from build123d import *

# Parameters (mm, degrees)
SKETCH1_W               = 61.1
SKETCH1_H               = 60
BOSS_EXTRUDE1_DEPTH     = 5
BOSS_EXTRUDE2_DEPTH     = 24
MIRROR2_COPY_1_DEPTH    = 24
SKETCH3_R               = 1.75
CUT_EXTRUDE1_DEPTH      = 60.592417722
MIRROR4_COPY_1_SKETCH_R = 1.75
MIRROR4_COPY_1_DEPTH    = 60.592417722
MIRROR5_COPY_1_SKETCH_R = 1.75
MIRROR5_COPY_1_DEPTH    = 60.592417722
MIRROR5_COPY_2_SKETCH_R = 1.75
MIRROR5_COPY_2_DEPTH    = 60.592417722
MIRROR5_COPY_3_SKETCH_R = 1.75
MIRROR5_COPY_3_DEPTH    = 60.592417722
SKETCH10_R              = 1.55
CUT_EXTRUDE7_DEPTH      = 8
SKETCH11_R              = 3
CUT_EXTRUDE8_DEPTH      = 1
SKETCH12_W              = 2
SKETCH12_H              = 30
SKETCH12_W_2            = 4
BOSS_EXTRUDE5_DEPTH     = 6.5
FILLET1_R               = 5
SKETCH12_4_W            = 0.75
SKETCH12_4_H            = 1
BOSS_EXTRUDE6_DEPTH     = 6.5
LPATTERN1_COUNT         = 15
LPATTERN1_PITCH         = 2
SKETCH13_R              = 1.55
CUT_EXTRUDE9_DEPTH      = 6.5


with BuildPart() as part:
    # Sketch1 → Boss-Extrude1 (new body)
    with BuildSketch(Plane(origin=(0, 0, 0), x_dir=(1, 0, 0), z_dir=(0, 1, 0))):
        Rectangle(SKETCH1_W, SKETCH1_H)
    extrude(amount=BOSS_EXTRUDE1_DEPTH)

    # Sketch2 → Boss-Extrude2 (add)
    with BuildSketch(Plane.XY.offset(30)):
        with BuildLine():
            Line((-30.55, 15.75), (-30.55, 5))
            Line((-30.55, 5), (-13.45, 5))
            Line((-13.45, 5), (-13.45, 15.75))
            Line((-13.45, 15.75), (-14.45, 15.75))
            ThreePointArc((-14.45, 15.75), (-22, 8.2), (-29.55, 15.75))
            Line((-29.55, 15.75), (-30.55, 15.75))
        make_face()
    boss_extrude2 = extrude(amount=-BOSS_EXTRUDE2_DEPTH)

    # Mirror1: Boss-Extrude2 across plane
    add(boss_extrude2.mirror(Plane.XY))

    # Mirror2: Boss-Extrude2 across plane
    add(boss_extrude2.mirror(Plane(origin=(0, 0, 0), x_dir=(0, 0, 1), z_dir=(1, 0, 0))))

    # Mirror2 copy 1 sketch → Mirror2 copy 1 (add)
    with BuildSketch(Plane(origin=(0, 0, -30), x_dir=(-1, 0, 0), z_dir=(0, 0, -1))):
        with BuildLine():
            Line((-30.55, 15.75), (-30.55, 5))
            Line((-30.55, 5), (-13.45, 5))
            Line((-13.45, 5), (-13.45, 15.75))
            Line((-13.45, 15.75), (-14.45, 15.75))
            ThreePointArc((-14.45, 15.75), (-22, 8.2), (-29.55, 15.75))
            Line((-29.55, 15.75), (-30.55, 15.75))
        make_face()
    extrude(amount=-MIRROR2_COPY_1_DEPTH)

    # Sketch3 → Cut-Extrude1 (cut, symmetric)
    with BuildSketch(Plane(origin=(-17.775, 17.775, 0), x_dir=(0.7071067811865477, 0.7071067811865475, 0), z_dir=(-0.7071067811865475, 0.7071067811865477, 0))):
        with Locations(Location((-13.965180362, -18, 0), (0, 0, 180))):
            Circle(SKETCH3_R)
    cut_extrude1 = extrude(amount=CUT_EXTRUDE1_DEPTH, both=True, mode=Mode.SUBTRACT)

    # Mirror3: Cut-Extrude1 across plane
    add(cut_extrude1.mirror(Plane.ZY.offset(22)), mode=Mode.SUBTRACT)

    # Mirror4: Cut-Extrude1 across plane
    add(cut_extrude1.mirror(Plane.XY), mode=Mode.SUBTRACT)

    # Mirror4 copy 1 sketch → Mirror4 copy 1 (cut, symmetric)
    with BuildSketch(Plane(origin=(-26.225, 17.775, 0), x_dir=(-0.7071067811865477, 0.7071067811865475, 0), z_dir=(0.7071067811865475, 0.7071067811865477, 0))):
        with Locations(Location((-13.965180362, -18, 0), (0, 0, 180))):
            Circle(MIRROR4_COPY_1_SKETCH_R)
    extrude(amount=MIRROR4_COPY_1_DEPTH, both=True, mode=Mode.SUBTRACT)

    # Mirror5: Cut-Extrude1 across plane
    add(cut_extrude1.mirror(Plane(origin=(0, 0, 0), x_dir=(0, 0, 1), z_dir=(1, 0, 0))), mode=Mode.SUBTRACT)

    # Mirror5 copy 1 sketch → Mirror5 copy 1 (cut, symmetric)
    with BuildSketch(Plane(origin=(26.225, 17.775, 0), x_dir=(0.7071067811865477, 0.7071067811865475, 0), z_dir=(-0.7071067811865475, 0.7071067811865477, 0))):
        with Locations(Location((-13.965180362, -18, 0), (0, 0, 180))):
            Circle(MIRROR5_COPY_1_SKETCH_R)
    extrude(amount=MIRROR5_COPY_1_DEPTH, both=True, mode=Mode.SUBTRACT)

    # Mirror5 copy 2 sketch → Mirror5 copy 2 (cut, symmetric)
    with BuildSketch(Plane(origin=(17.775, 17.775, 0), x_dir=(-0.7071067811865477, 0.7071067811865475, 0), z_dir=(0.7071067811865475, 0.7071067811865477, 0))):
        with Locations(Location((-13.965180362, -18, 0), (0, 0, 180))):
            Circle(MIRROR5_COPY_2_SKETCH_R)
    extrude(amount=MIRROR5_COPY_2_DEPTH, both=True, mode=Mode.SUBTRACT)

    # Mirror5 copy 3 sketch → Mirror5 copy 3 (cut, symmetric)
    with BuildSketch(Plane(origin=(26.225, 17.775, 0), x_dir=(0.7071067811865477, 0.7071067811865475, 0), z_dir=(-0.7071067811865475, 0.7071067811865477, 0))):
        with Locations((-13.965180362, 18)):
            Circle(MIRROR5_COPY_3_SKETCH_R)
    extrude(amount=MIRROR5_COPY_3_DEPTH, both=True, mode=Mode.SUBTRACT)

    # Sketch10 → Cut-Extrude7 (cut)
    with BuildSketch(Plane(origin=(0, 5, 0), x_dir=(1, 0, 0), z_dir=(0, 1, 0))):
        with Locations(Location((-6.45, -26, 0), (0, 0, 270))):
            Circle(SKETCH10_R)
        with Locations(Location((-6.45, 26, 0), (0, 0, 270))):
            Circle(SKETCH10_R)
        with Locations(Location((6.45, 26, 0), (0, 0, 270))):
            Circle(SKETCH10_R)
        with Locations(Location((6.45, -26, 0), (0, 0, 270))):
            Circle(SKETCH10_R)
    extrude(amount=-CUT_EXTRUDE7_DEPTH, mode=Mode.SUBTRACT)

    # Sketch11 → Cut-Extrude8 (cut)
    with BuildSketch(Plane.XZ):
        with Locations(Location((-6.45, 26, 0), (0, 0, 270))):
            Circle(SKETCH11_R)
        with Locations(Location((6.45, 26, 0), (0, 0, 270))):
            Circle(SKETCH11_R)
        with Locations(Location((6.45, -26, 0), (0, 0, 270))):
            Circle(SKETCH11_R)
        with Locations(Location((-6.45, -26, 0), (0, 0, 270))):
            Circle(SKETCH11_R)
    extrude(amount=-CUT_EXTRUDE8_DEPTH, mode=Mode.SUBTRACT)

    # Sketch12 → Boss-Extrude5 (add)
    with BuildSketch(Plane(origin=(0, 5, 0), x_dir=(1, 0, 0), z_dir=(0, 1, 0))):
        with Locations((-13.45, 0)):
            Rectangle(SKETCH12_W, SKETCH12_H)
        with Locations((-8.85, 0)):
            Rectangle(SKETCH12_W_2, SKETCH12_H)
    extrude(amount=BOSS_EXTRUDE5_DEPTH)

    # Fillet1
    fillet1_edges = [part.edges().sort_by_distance(p)[0] for p in [
        (-8.85, 5, 15),
        (-6.85, 5, 0),
        (-8.85, 5, -15),
        (-12.95, 5, -15),
        (-14.45, 5, 0),
        (-12.95, 5, 15),
    ]]
    fillet(fillet1_edges, radius=FILLET1_R)

    # Sketch12_4 → Boss-Extrude6 (add)
    with BuildSketch(Plane(origin=(0, 5, 0), x_dir=(1, 0, 0), z_dir=(0, 1, 0))):
        with Locations((-11.225, 14.5)):
            Rectangle(SKETCH12_4_W, SKETCH12_4_H)
    boss_extrude6 = extrude(amount=BOSS_EXTRUDE6_DEPTH)

    # LPattern1: Boss-Extrude6 ×15
    with Locations(*[(0, 0, i * LPATTERN1_PITCH) for i in range(1, LPATTERN1_COUNT)]):
        add(boss_extrude6)

    # Sketch13 → Cut-Extrude9 (cut)
    with BuildSketch(Plane.XZ):
        with Locations(Location((0, 10, 0), (0, 0, 270))):
            Circle(SKETCH13_R)
        with Locations(Location((0, -10, 0), (0, 0, 270))):
            Circle(SKETCH13_R)
    extrude(amount=-CUT_EXTRUDE9_DEPTH, mode=Mode.SUBTRACT)


solid = part.part
Check sheet for the modelled part. Datum: model origin and axes. Units: mm. A direction names the side the tool comes from. Coordinates: 2 decimals unless noted, no trailing zeros. Loops run counter-clockwise (first coordinate to the right, second up) from the corner with the lowest first, then second, coordinate; pieces in that order, holes last. Notation, with made-up numbers: (81.25, 48.25) -> (113.25, 48.25) arc R9 cw to (113.25, 54.25) -> close; hole circle Ø6 at (-29.75, -18.75). An arc over 180 degrees is marked (long way). Answer in a Markdown table with one row per item.
1. Material ranges on line 1 along X through (y, z) = (3.6, -26); line 2 along X through (y, z) = (0.7, 26); line 3 along X through (y, z) = (15.25, -22), recorded low to high. Write a range as [from, to].
Check values:
| item | result |
|---|---|
| line 1 | x = [-30.55, -8], [-4.9, 4.9], [8, 30.55] |
| line 2 | x = [-30.55, -9.45], [-3.45, 3.45], [9.45, 30.55] |
| line 3 | x = [-30.55, -29.53], [-14.47, -13.45], [13.45, 14.47], [29.53, 30.55] |
2. Access from +Z, -Z, +X, -X, +Y, -Y to the whole of each face (thin tool, end or side, straight path). Record for faces 4 (the face through (-9, 11, 15)), 5 (the face through (5, 1, -27)), 6 (the face through (13.45, 8, -18)), 7 (the face through (22, 8, 6)).
Check values:
| item | result |
|---|---|
| face 4 | +Z, +Y |
| face 5 | -Y |
| face 6 | +Z, -Z, +Y |
| face 7 | +X, +Y |
3. Sectioned sample at A-A, the plane x = 6.45. Record the boundary of the cut face in (y, z).
Check values:
| item | result |
|---|---|
| outline | (0, -30) -> (5, -30) -> (5, -27.55) -> (1, -27.55) -> (1, -29) -> (0, -29) -> close; (0, -23) -> (1, -23) -> (1, -24.45) -> (5, -24.45) -> (5, 24.45) -> (1, 24.45) -> (1, 23) -> (0, 23) -> close; (0, 29) -> (1, 29) -> (1, 27.55) -> (5, 27.55) -> (5, 30) -> (0, 30) -> close |
4. Sectioned sample at C-C, the plane x = 0. Record the boundary of the cut face in (y, z).
Check values:
| item | result |
|---|---|
| outline | (0, -30) -> (5, -30) -> (5, -11.55) -> (0, -11.55) -> close; (0, -8.45) -> (5, -8.45) -> (5, 8.45) -> (0, 8.45) -> close; (0, 11.55) -> (5, 11.55) -> (5, 30) -> (0, 30) -> close |
5. Go/stop test with flat-tipped pins: pin 1 (4 mm diameter, centred on y = 11, z = 3, fed in from -X); pin 2 (0.8 mm diameter, centred on y = 7.5, z = 5.5, fed in from -X); pin 3 (0.8 mm diameter, centred on x = -11.5, y = 7.5, fed in from -Z). Record where each tip stops, or that it passes through.
Check values:
| item | result |
|---|---|
| pin 1 | stops at x = -14.55 |
| pin 2 | stops at x = -15.38 |
| pin 3 | stops at z = -15 |
6. Release check for a two-part mould opening along Y. For faces 1 (the face through (-8, 1, 25)), 2 (the face through (18.987, 1.71, 18.066)), 3 (the face through (0, 4, 30)) record: released by +Y, released by -Y, zero draft, split by the parting line, or undercut.
Check values:
| item | result |
|---|---|
| face 1 | released by -Y |
| face 2 | undercut |
| face 3 | zero draft |
7. Sectioned sample at B-B, the plane y = 7.5. Give the number of separate pieces and of enclosed holes in the cut face, then the cut area to 3 significant figures.
Check values:
| item | result |
|---|---|
| separate pieces | 4 |
| enclosed holes | 8 |
| area | 1,740 mm2 |
